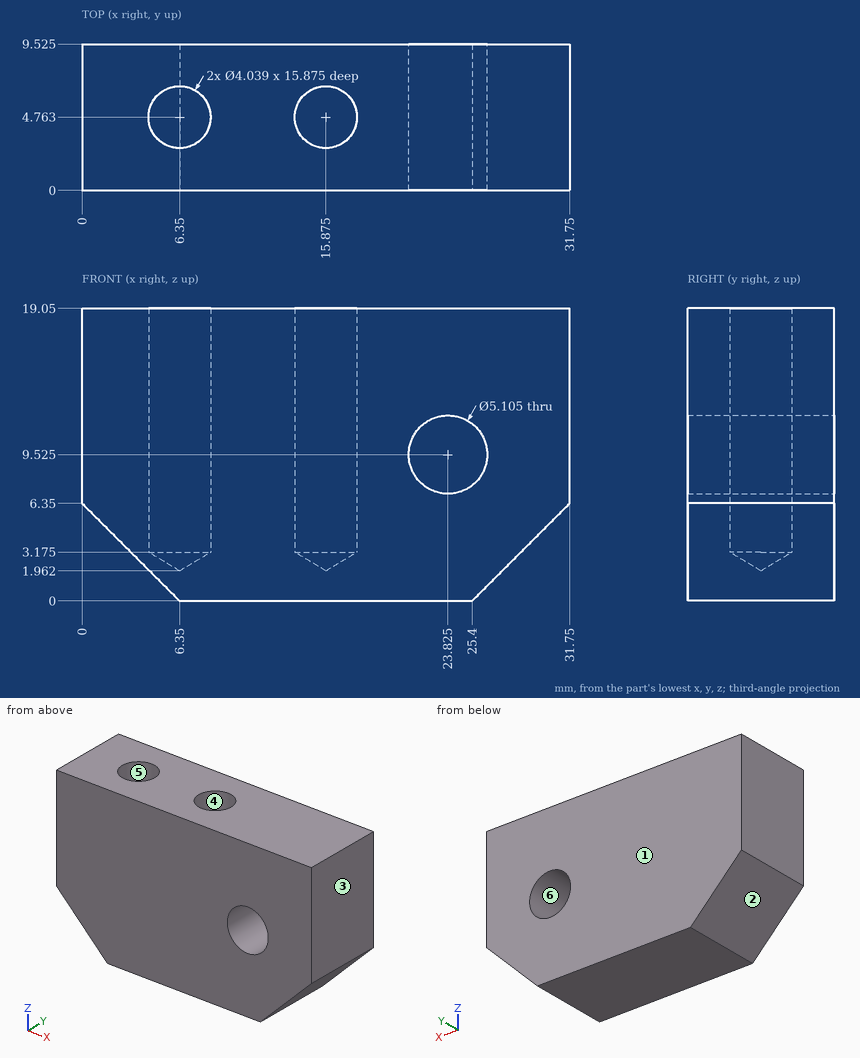
Source: three-view drawing plus pictorial views. Frame: mm from the lowest corner of the part. A direction names the side the tool comes from. Round coordinates to 2 decimals unless told otherwise and drop trailing zeros. Answer in a Markdown table with one row per item.
Item 1: Line query: line 1 (Y direction, x = 6.35, z = 7.5) (1 decimal); line 2 (Y direction, x = 17.5, z = 8) (1 decimal); line 3 (X direction, y = 8, z = 9). Output: solid intervals per line, ascending.
Model answer:
| item | result |
|---|---|
| line 1 | y = 0 to 2.7, 6.8 to 9.5 |
| line 2 | y = 0 to 3.6, 6 to 9.5 |
| line 3 | x = 0 to 21.33, 26.32 to 31.75 |
Item 2: Mould query, pull axis X, two halves, no side actions, for the marked faces 1, 2, 3 and 4. Classes: released by +X, released by -X, zero draft, split by the parting line, or undercut.
Model answer:
| item | result |
|---|---|
| face 1 | zero draft |
| face 2 | released by -X |
| face 3 | released by +X |
| face 4 | undercut |
Item 3: Reachability of the marked faces 5 and 6 from +Z, -Z, +X, -X, +Y, -Y: full face, straight path, thin tool, end or side. Return the list, or none.
Model answer:
| item | result |
|---|---|
| face 5 | +Z |
| face 6 | +Y, -Y |
